```python
from build123d import *

# Parameters (mm, degrees)
F0_W     = 117.2845363617
F0_H     = 97.3939225078
F1_DEPTH = 40
F2_R     = 9
F4_R     = 30.8763163617
F5_DEPTH = 25.4
F6_DEPTH = 25.4


with BuildPart() as f1:
    # F0 (on Front) → F1 (new body)
    with BuildSketch(Plane.XZ):
        Rectangle(F0_W, F0_H)
    extrude(amount=F1_DEPTH)

    # F2
    f2_edges = [f1.edges().sort_by_distance(p)[0] for p in [
        (0, 0, 48.696961),
        (0, -40, 48.696961),
        (0, -40, -48.696961),
        (0, 0, -48.696961),
    ]]
    fillet(f2_edges, radius=F2_R)

    # F4 (on face) → F5 (join)
    with BuildSketch(Plane.XZ.offset(40)):
        Circle(F4_R)
    extrude(amount=F5_DEPTH)

    # F6 (add): a face of the model
    f6_faces = [f1.faces().sort_by_distance(p)[0] for p in [
        (0, 0, 0),
    ]]
    extrude(f6_faces, amount=F6_DEPTH)


solid = f1.part
```
Geometry: final body of the model. Coordinates: model frame, mm. A direction names the side the tool comes from. Coordinates: 2 decimals unless noted, no trailing zeros. Order: outer loops, then holes, each group sorted by start corner. A loop starts at its lowest first (then second) coordinate and runs counter-clockwise, first axis right, second up. Notation, with made-up numbers: (-16.75, -29.5) -> (40.25, -29.5) arc R30 ccw to (40.25, -2.5) -> close; hole circle Ø3 at (-13, 77). An arc over 180 degrees is marked (long way). Write each question's results on one line, items separated by ' | '. Start each with the question number.
1) Cut plane C-C, the plane y = -49.5. Output: boundary loops of the cut face in (x, z).
2) Cut plane A-A, the plane x = 0. Output: boundary loops of the cut face in (y, z).
3) Material intervals for line 1 along Y through (x, z) = (7.5, -39.5); line 2 along Z through (x, y) = (-6.5, 6.5); line 3 along Y through (x, z) = (-5, 40.5), sorted ascending.
4) First-contact query: pin 1 (20.5 mm diameter, centred on x = -25.5, y = 6.5, fed in from +Z); pin 2 (1 mm diameter, centred on y = -53, z = 27.5, fed in from +X); pin 3 (8 mm diameter, centred on x = -25.5, y = -7.5, fed in from +Z); pin 4 (20.5 mm diameter, centred on x = 23.5, y = 10.5, fed in from -Z). Flat tips, straight axial feed; report the tip coordinate or a pass-through.
5) Set-up query: faces 1 (the flat face through (0, -65.4, 0)), 2 (the flat face through (-1, 13, -39.697)), 3 (the cylindrical face through (-24.5, -52.52, -18.79)), 4 (the flat face through (-1, 13, 39.697)). Return all of +Z, -Z, +X, -X, +Y, -Y with unobstructed straight access to the full face (end or side cutting, diameter ignored); none if empty.
6) Cut plane D-D, the plane z = -10.5. Output: boundary loops of the cut face in (x, y), and give its area (3 significant figures).
7) Cut plane B-B, the plane z = 0. Output: boundary loops of the cut face in (x, y).
Checks:
1) outline: circle Ø61.75 at (0, 0)
2) outline: (-65.4, -30.88) -> (-40, -30.88) -> (-40, -39.7) arc R9 ccw to (-31, -48.7) -> (-9, -48.7) arc R9 ccw to (0, -39.7) -> (25.4, -39.7) -> (25.4, 39.7) -> (0, 39.7) arc R9 ccw to (-9, 48.7) -> (-31, 48.7) arc R9 ccw to (-40, 39.7) -> (-40, 30.88) -> (-65.4, 30.88) -> close
3) line 1: -40 to 25.4 | line 2: -39.7 to 39.7 | line 3: -39.96 to -0.04
4) pin 1: z = 47.01 | pin 2: x = 14.98 | pin 3: z = 48.7 | pin 4: z = -39.7
5) face 1: +Z, -Z, +X, -X, -Y | face 2: -Z, +X, -X, +Y | face 3: -Y | face 4: +Z, +X, -X, +Y
6) outline: (-58.64, -40) -> (-29.04, -40) -> (-29.04, -65.4) -> (29.04, -65.4) -> (29.04, -40) -> (58.64, -40) -> (58.64, 25.4) -> (-58.64, 25.4) -> close | area: 9,150 mm^2
7) outline: (-58.64, -40) -> (-30.88, -40) -> (-30.88, -65.4) -> (30.88, -65.4) -> (30.88, -40) -> (58.64, -40) -> (58.64, 25.4) -> (-58.64, 25.4) -> close
